```python
from build123d import *

# Parameters (mm, degrees)
BOSS_EXTRUDE1_DEPTH        = 6
BOSS_EXTRUDE1_DEPTH_BACK   = 2.5
SKETCH1_R                  = 2.5
SKETCH1_R_2                = 1.5
BOSS_EXTRUDE1_2_DEPTH      = 6
BOSS_EXTRUDE1_2_DEPTH_BACK = 2.5
BOSS_EXTRUDE1_3_DEPTH      = 6
BOSS_EXTRUDE1_3_DEPTH_BACK = 2.5
BOSS_EXTRUDE1_4_DEPTH      = 6
BOSS_EXTRUDE1_4_DEPTH_BACK = 2.5
SKETCH2_W                  = 50
SKETCH2_H                  = 42
BOSS_EXTRUDE3_DEPTH        = 4
CUT_EXTRUDE2_DEPTH         = 41.142251143
CUT_EXTRUDE2_DEPTH_BACK    = 41.142251143
SKETCH4_W                  = 26
SKETCH4_H                  = 32
BOSS_EXTRUDE4_DEPTH        = 3.5
BOSS_EXTRUDE4_DEPTH_BACK   = 4
SKETCH5_W                  = 3
SKETCH5_H                  = 22
BOSS_EXTRUDE5_DEPTH        = 3.5
BOSS_EXTRUDE5_DEPTH_BACK   = 4
SKETCH6_W                  = 12
SKETCH6_H                  = 3
SKETCH3_R                  = 1.5
CUT_EXTRUDE3_DEPTH         = 6
BOSS_EXTRUDE6_START        = -4
BOSS_EXTRUDE6_DEPTH        = 4
CUT_EXTRUDE6_DEPTH         = 4
FILLET1_R                  = 1
FILLET2_R                  = 1
FILLET3_R                  = 1
FILLET4_R                  = 1


# Read off the part's stored shape, not the designer's step: Boss-Extrude6
with BuildPart() as part:
    # Sketch1 → Boss-Extrude1 (new, two sides: drawn at the far end of the back side and taken through both)
    with BuildSketch(Plane(origin=(0, 0, 0), x_dir=(1, 0, 0), z_dir=(0, 1, 0)).offset(-BOSS_EXTRUDE1_DEPTH_BACK)):
        with Locations(Location((-21.137254902, 20.117647059, 0), (0, 0, 270))):
            Circle(SKETCH1_R)
        with Locations(Location((-21.137254902, 20.117647059, 0), (0, 0, 270))):
            Circle(SKETCH1_R_2, mode=Mode.SUBTRACT)
    extrude(amount=BOSS_EXTRUDE1_DEPTH + BOSS_EXTRUDE1_DEPTH_BACK)



with BuildPart() as body_2:
    # Sketch1 → Boss-Extrude1 2 (new, two sides: drawn at the far end of the back side and taken through both)
    with BuildSketch(Plane(origin=(0, 0, 0), x_dir=(1, 0, 0), z_dir=(0, 1, 0)).offset(-BOSS_EXTRUDE1_2_DEPTH_BACK)):
        with Locations(Location((11.862745098, 20.117647059, 0), (0, 0, 270))):
            Circle(SKETCH1_R)
        with Locations(Location((11.862745098, 20.117647059, 0), (0, 0, 270))):
            Circle(SKETCH1_R_2, mode=Mode.SUBTRACT)
    extrude(amount=BOSS_EXTRUDE1_2_DEPTH + BOSS_EXTRUDE1_2_DEPTH_BACK)


with BuildPart() as body_3:
    # Sketch1 → Boss-Extrude1 3 (new, two sides: drawn at the far end of the back side and taken through both)
    with BuildSketch(Plane(origin=(0, 0, 0), x_dir=(1, 0, 0), z_dir=(0, 1, 0)).offset(-BOSS_EXTRUDE1_3_DEPTH_BACK)):
        with Locations(Location((-21.137254902, -12.132352941, 0), (0, 0, 270))):
            Circle(SKETCH1_R)
        with Locations(Location((-21.137254902, -12.132352941, 0), (0, 0, 270))):
            Circle(SKETCH1_R_2, mode=Mode.SUBTRACT)
    extrude(amount=BOSS_EXTRUDE1_3_DEPTH + BOSS_EXTRUDE1_3_DEPTH_BACK)


with BuildPart() as body_4:
    # Sketch1 → Boss-Extrude1 4 (new, two sides: drawn at the far end of the back side and taken through both)
    with BuildSketch(Plane(origin=(0, 0, 0), x_dir=(1, 0, 0), z_dir=(0, 1, 0)).offset(-BOSS_EXTRUDE1_4_DEPTH_BACK)):
        with Locations(Location((11.862745098, -12.132352941, 0), (0, 0, 270))):
            Circle(SKETCH1_R)
        with Locations(Location((11.862745098, -12.132352941, 0), (0, 0, 270))):
            Circle(SKETCH1_R_2, mode=Mode.SUBTRACT)
    extrude(amount=BOSS_EXTRUDE1_4_DEPTH + BOSS_EXTRUDE1_4_DEPTH_BACK)


with BuildPart() as part_1:
    add(part.part)

    add(body_2.part)  # Boss-Extrude3 merges body 2

    add(body_3.part)  # Boss-Extrude3 merges body 3

    add(body_4.part)  # Boss-Extrude3 merges body 4
    # Sketch2 → Boss-Extrude3 (add)
    with BuildSketch(Plane(origin=(0, 6, 0), x_dir=(1, 0, 0), z_dir=(0, 1, 0))):
        with Locations((-5.137254902, 4.117647059)):
            Rectangle(SKETCH2_W, SKETCH2_H)
    extrude(amount=-BOSS_EXTRUDE3_DEPTH)

    # Sketch4 → Cut-Extrude2 (cut, two sides: drawn at the far end of the back side and taken through both)
    with BuildSketch(Plane(origin=(0, 6, 0), x_dir=(1, 0, 0), z_dir=(0, 1, 0)).offset(-CUT_EXTRUDE2_DEPTH_BACK)):
        with Locations((-4.637254902, 4.117647059)):
            Rectangle(SKETCH4_W, SKETCH4_H)
    extrude(amount=CUT_EXTRUDE2_DEPTH + CUT_EXTRUDE2_DEPTH_BACK, mode=Mode.SUBTRACT)

    # Sketch5 → Boss-Extrude4 (add, two sides: drawn at the far end of the back side and taken through both)
    with BuildSketch(Plane.XZ.offset(-2).offset(-BOSS_EXTRUDE4_DEPTH_BACK)):
        with Locations((21.362745098, -4.117647059)):
            Rectangle(SKETCH5_W, SKETCH5_H)
    extrude(amount=BOSS_EXTRUDE4_DEPTH + BOSS_EXTRUDE4_DEPTH_BACK)

    # Sketch6 → Boss-Extrude5 (add, two sides: drawn at the far end of the back side and taken through both)
    with BuildSketch(Plane.XZ.offset(-2).offset(-BOSS_EXTRUDE5_DEPTH_BACK)):
        with Locations((-3.137254902, -26.617647059)):
            Rectangle(SKETCH6_W, SKETCH6_H)
    extrude(amount=BOSS_EXTRUDE5_DEPTH + BOSS_EXTRUDE5_DEPTH_BACK)

    # Sketch3 → Cut-Extrude3 (cut)
    with BuildSketch(Plane(origin=(0, 6, 0), x_dir=(1, 0, 0), z_dir=(0, 1, 0))):
        with Locations(Location((-21.137254902, 20.117647059, 0), (0, 0, 270))):
            Circle(SKETCH3_R)
        with Locations(Location((-21.137254902, -12.132352941, 0), (0, 0, 270))):
            Circle(SKETCH3_R)
        with Locations(Location((11.862745098, -12.132352941, 0), (0, 0, 270))):
            Circle(SKETCH3_R)
        with Locations(Location((11.862745098, 20.117647059, 0), (0, 0, 270))):
            Circle(SKETCH3_R)
    extrude(amount=-CUT_EXTRUDE3_DEPTH, mode=Mode.SUBTRACT)

    # Sketch10 → Cut-Extrude6 (cut)
    with BuildSketch(Plane(origin=(0, 6, 0), x_dir=(1, 0, 0), z_dir=(0, 1, 0))):
        Polygon((8.362745098, 20.117647059), (12.362745098, 25.117647059), (-21.637254902, 25.117647059), (-17.637254902, 20.117647059), align=None)
        Polygon((-17.637254902, -11.882352941), (-21.637254902, -16.882352941), (12.362745098, -16.882352941), (8.362745098, -11.882352941), align=None)
    extrude(amount=-CUT_EXTRUDE6_DEPTH, mode=Mode.SUBTRACT)


with BuildPart() as body_2_2:
    # Boss-Extrude6 outline → Boss-Extrude6 (new body)
    with BuildSketch(Plane(origin=(0, 6, 0), x_dir=(1, 0, 0), z_dir=(0, 1, 0)).offset(BOSS_EXTRUDE6_START)):
        Polygon((-9.137254902, 25.117647059), (-9.137254902, 28.117647059), (-33.137254902, 28.117647059), (-33.137254902, -19.882352941), (22.862745098, -19.882352941), (22.862745098, -6.882352941), (19.862745098, -6.882352941), (19.862745098, -16.882352941), (-30.137254902, -16.882352941), (-30.137254902, 25.117647059), align=None)
        Polygon((22.862745098, 28.117647059), (2.862745098, 28.117647059), (2.862745098, 25.117647059), (19.862745098, 25.117647059), (19.862745098, 15.117647059), (22.862745098, 15.117647059), align=None)
    extrude(amount=BOSS_EXTRUDE6_DEPTH)


with BuildPart() as cut_extrude6_piece_1:
    # of the separate pieces the step leaves, piece 1, a body of its own (cut_extrude6_pieces)
    add(part_1.part.solids().sort_by_distance((8.362745098, 2, -20.117647059))[0])

    # Fillet2
    fillet2_edges = [cut_extrude6_piece_1.edges().sort_by_distance(p)[0] for p in [
        (8.362745098, 4, 11.882352941),
        (8.362745098, 4, -20.117647059),
    ]]
    fillet(fillet2_edges, radius=FILLET2_R)

    # Fillet4
    fillet4_edges = [cut_extrude6_piece_1.edges().sort_by_distance(p)[0] for p in [
        (21.362745098, -1.5, -15.117647059),
        (21.362745098, -1.5, 6.882352941),
    ]]
    fillet(fillet4_edges, radius=FILLET4_R)


with BuildPart() as cut_extrude6_piece_2:
    # of the separate pieces the step leaves, piece 2, a body of its own (cut_extrude6_pieces)
    add(part_1.part.solids().sort_by_distance((-21.137254902, 0, -17.617647059))[0])

    # Fillet1
    fillet1_edges = [cut_extrude6_piece_2.edges().sort_by_distance(p)[0] for p in [
        (-17.637254902, 4, 11.882352941),
        (-17.637254902, 4, -20.117647059),
    ]]
    fillet(fillet1_edges, radius=FILLET1_R)


with BuildPart() as cut_extrude6_piece_3:
    # of the separate pieces the step leaves, piece 3, a body of its own (cut_extrude6_pieces)
    add(part_1.part.solids().sort_by_distance((-9.137254902, -1.5, -25.117647059))[0])

    # Fillet3
    fillet3_edges = [cut_extrude6_piece_3.edges().sort_by_distance(p)[0] for p in [
        (-9.137254902, -1.5, -26.617647059),
        (2.862745098, -1.5, -26.617647059),
    ]]
    fillet(fillet3_edges, radius=FILLET3_R)


with BuildPart() as body_2_2_1:
    add(body_2_2.part)

    # Combine1: union Cut-Extrude6 piece 2, Cut-Extrude6 piece 3, Cut-Extrude6 piece 1
    add(cut_extrude6_piece_2.part)
    add(cut_extrude6_piece_3.part)
    add(cut_extrude6_piece_1.part)


solid = body_2_2_1.part
```
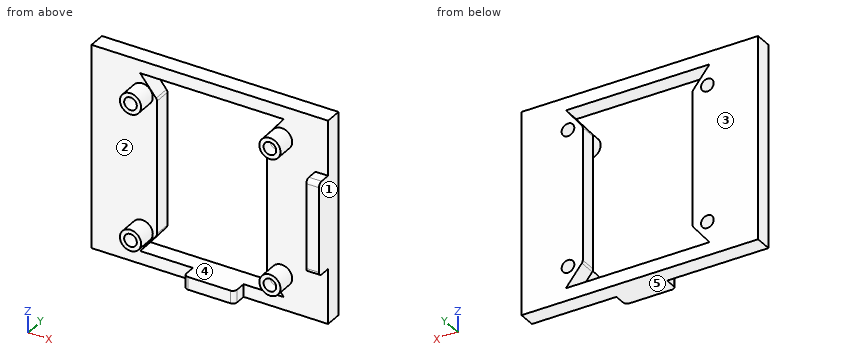
Source: CAD feature listing. Evaluate the final solid. Frame: model axes, mm. Face numbers are marked on the shaded views. A direction names the side the tool comes from. Round coordinates to 2 decimals unless told otherwise and drop trailing zeros. Order: outer loops, then holes, each group sorted by start corner. A loop starts at its lowest first (then second) coordinate and runs counter-clockwise, first axis right, second up. Notation, with made-up numbers: (22, -29.5) -> (35, -29.5) arc R26 cw to (35, -11.5) -> close; hole circle Ø5 at (83.5, 86.5). An arc over 180 degrees is marked (long way). Use CSV: the item, a comma, the result in double quotes.
(1) First-contact query: pin 1 Ø2.5 at (x, z) = (-21.14, -20.12) entering from +Y; pin 2 Ø4 at (x, z) = (11.86, 12.13) entering from +Y; pin 3 Ø0.8 at (x, y) = (21, 1) entering from -Z; pin 4 Ø2.5 at (x, z) = (21.5, -0.5) entering from -Y. Flat tips, straight axial feed; report the tip coordinate or a pass-through.
Report:
pin 1,"through"
pin 2,"y = 6"
pin 3,"z = -15.12"
pin 4,"y = -1.5"
(2) Ray query, L1, parallel to X at y = 5.25, z = 10; L2, parallel to Z at x = 12, y = 3; L3, parallel to Z at x = 1.5, y = 2.75. Return the intervals inside material, ascending.
Report:
L1,"-33.14 to -17.64, 8.36 to 22.86"
L2,"-28.12 to -25.12, -24.66 to -21.61, -18.62 to 10.64, 13.63 to 16.43, 16.88 to 19.88"
L3,"-28.12 to -25.12, 16.88 to 19.88"
(3) Section B-B on z = -5.5. Return the cut outline in (x, y).
Report:
outline,"(-33.14, 2) -> (-17.64, 2) -> (-17.64, 6) -> (-33.14, 6) -> close; (8.36, 2) -> (19.86, 2) -> (19.86, -1.5) -> (22.86, -1.5) -> (22.86, 6) -> (8.36, 6) -> close"
(4) Access query for the marked faces 1 and 2. Directions: +Z, -Z, +X, -X, +Y, -Y. A direction counts if a zero-diameter tool reaches every point of the face in a straight line with its end or side. Return the directions, or none.
Report:
face 1,"+Z, -Z, +X, +Y, -Y"
face 2,"-Y"
(5) Section C-C on y = 3.25. Return the cut outline in (x, z), and give its area (3 significant figures).
Report:
outline,"(-33.14, -28.12) -> (22.86, -28.12) -> (22.86, 19.88) -> (-33.14, 19.88) -> close; hole circle Ø3 at (-21.14, -20.12); hole circle Ø3 at (-21.14, 12.13); hole (-21.64, -25.12) -> (12.36, -25.12) -> (8.58, -20.39) arc R1 cw to (8.36, -19.77) -> (8.36, 11.53) arc R1 cw to (8.58, 12.16) -> (12.36, 16.88) -> (-21.64, 16.88) -> (-17.86, 12.16) arc R1 cw to (-17.64, 11.53) -> (-17.64, -19.77) arc R1 cw to (-17.86, -20.39) -> close; hole circle Ø3 at (11.86, -20.12); hole circle Ø3 at (11.86, 12.13)"
area,"1,530 mm^2"
(6) Section A-A on x = -7. Return the cut outline in (y, z).
Report:
outline,"(-1.5, -28.12) -> (6, -28.12) -> (6, -25.12) -> (-1.5, -25.12) -> close; (2, 16.88) -> (6, 16.88) -> (6, 19.88) -> (2, 19.88) -> close"
(7) Pull-direction query (Z, two-part tool) for the marked faces 3, 4 and 5; classes: +Z half, -Z half, draft (parallel to the pull), parting line (faces both ways), or undercut.
Report:
face 3,"draft"
face 4,"undercut"
face 5,"-Z half"
(8) Section D-D on x = 7.5. Return the cut outline in (y, z), and give its area (3 significant figures).
Report:
outline,"(2, -28.12) -> (6, -28.12) -> (6, -25.12) -> (2, -25.12) -> close; (2, 16.88) -> (6, 16.88) -> (6, 19.88) -> (2, 19.88) -> close"
area,"24.0 mm^2"
